Drawing for the job (mm, zero at the part's lowest x, y, z). Give positions to 0.01 mm unless a question says otherwise; leave off trailing zeros. Loops run counter-clockwise (first coordinate to the right, second up) from the corner with the lowest first, then second, coordinate; pieces in that order, holes last.
1) Flat gauge pins, fed straight in: P1, Ø6.5, axis at x = 21.45, y = 21.45, coming from the +Z side; P2, Ø4, axis at x = 68.55, y = 21.45, coming from the -Z side. Where does each tip first touch, or does it go through?
2) Two-plate mould, pull along X, no slides. Class the marked faces 1 and 2: +X half, -X half, draft (parallel to the pull), parting line (faces both ways), or undercut.
3) Band-saw the part on D-D on z = 81. List the corners of the cut face in (x, y).
4) Band-saw the part on A-A on y = 68.55. List the corners of the cut face in (x, z), then the cut area to 3 significant figures.
5) Band-saw the part on B-B on y = 84. State how many separate pieces and enclosed holes the cut face has.
6) Wall check: line 1 (Y direction, x = 6.5, z = 159); line 2 (Y direction, x = 85, z = 65.5); line 3 (Z direction, x = 52.5, y = 83) (1 decimal). Give the ranges that are in metal, low to high.
7) Band-saw the part on C-C on x = 9.5. List the corners of the cut face in (y, z).
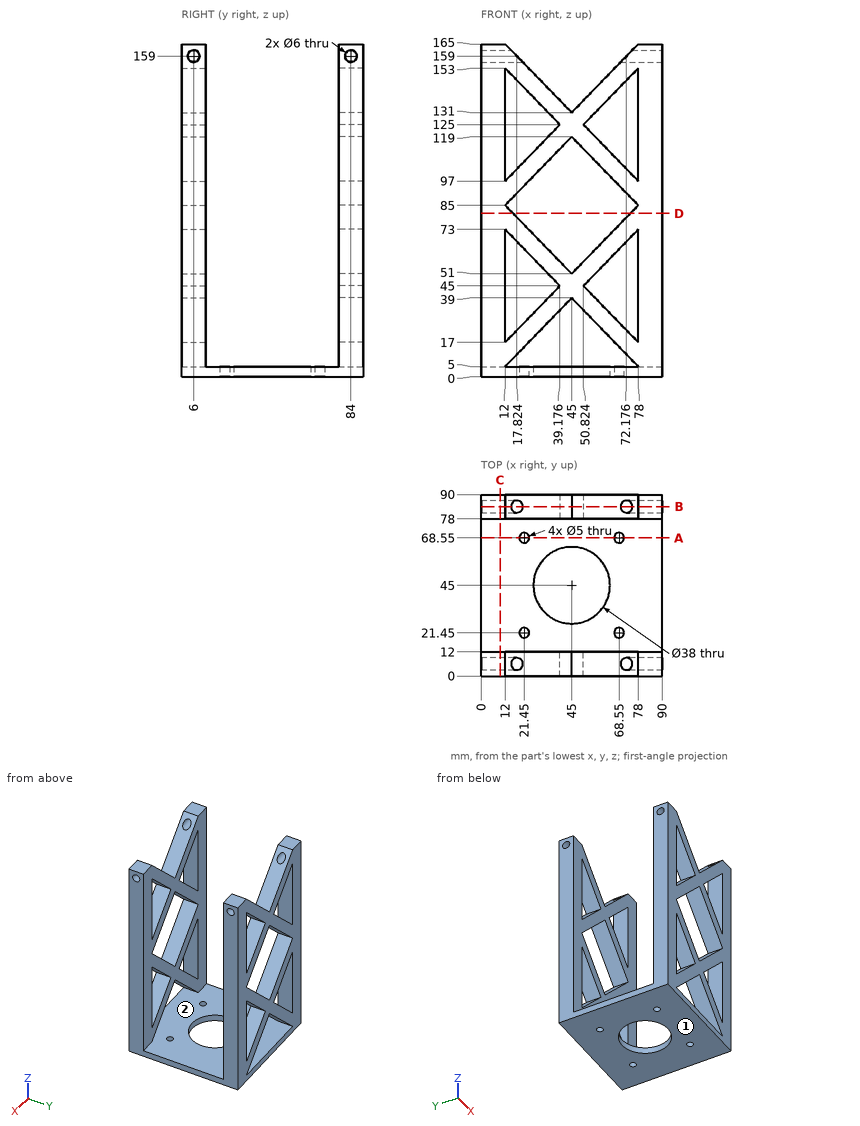
Findings below:
1. P1: stops at z = 5
1. P2: passes through
2. face 1: draft
2. face 2: undercut
3. outline: (0, 0) - (15.88, 0) - (15.88, 12) - (0, 12) - close; (0, 78) - (15.88, 78) - (15.88, 90) - (0, 90) - close; (74.12, 0) - (90, 0) - (90, 12) - (74.12, 12) - close; (74.12, 78) - (90, 78) - (90, 90) - (74.12, 90) - close
4. outline: (0, 0) - (18.95, 0) - (18.95, 5) - (0, 5) - close; (23.95, 0) - (66.05, 0) - (66.05, 5) - (23.95, 5) - close; (71.05, 0) - (90, 0) - (90, 5) - (71.05, 5) - close
4. area: 400 mm2
5. separate pieces: 3
5. enclosed holes: 6
6. line 1: y = 0 to 3, 9 to 12, 78 to 81, 87 to 90
6. line 2: y = 0 to 12, 78 to 90
6. line 3: z = 0 to 5, 31.3 to 43.3, 46.7 to 58.7, 111.3 to 123.3, 126.7 to 138.7
7. outline: (0, 0) - (90, 0) - (90, 165) - (78, 165) - (78, 5) - (12, 5) - (12, 165) - (0, 165) - close; hole circle Ø6 at (6, 159); hole circle Ø6 at (84, 159)
